from build123d import *

# Parameters (mm, degrees)
ESQUISSE1_R      = 28.5
EXTRUSION1_DEPTH = 5
ESQUISSE2_R      = 7.5
EXTRUSION2_DEPTH = 5
EXTRUSION3_REACH = 43.527
ESQUISSE3_R      = 2.5
ESQUISSE12_W     = 1.25
ESQUISSE12_H     = 28.5


with BuildPart() as part:
    # Esquisse1 → Extrusion1 (new body)
    with BuildSketch(Plane.XY):
        Circle(ESQUISSE1_R)
    extrude(amount=-EXTRUSION1_DEPTH)

    # Esquisse2 → Extrusion2 (add)
    with BuildSketch(Plane.XY):
        Circle(ESQUISSE2_R)
    extrude(amount=EXTRUSION2_DEPTH)

    # Esquisse3 → Extrusion3 (cut, up to next)
    with BuildSketch(Plane.XY.offset(5), mode=Mode.PRIVATE) as extrusion3_sk1:
        Circle(ESQUISSE3_R)
    extrusion3_tool1 = extrude(extrusion3_sk1.sketch, amount=-EXTRUSION3_REACH, mode=Mode.PRIVATE) & part.part
    add(extrusion3_tool1.solids().sort_by_distance((0, 0, 5))[0], mode=Mode.SUBTRACT)

    # Esquisse6 → Enlèvement de matière-Révolution3 (revolve, cut)
    with BuildSketch(Plane(origin=(0, 0, 0), x_dir=(1, 0, 0), z_dir=(0, 1, 0)), mode=Mode.PRIVATE) as enl_vement_de_mati_re_r_volution3_sk:
        with BuildLine():
            Line((-29, 4.5), (-31.449617094, 4.5))
            Line((-31.449617094, 4.5), (-31.449617094, 0.5))
            Line((-31.449617094, 0.5), (-29, 0.5))
            ThreePointArc((-29, 0.5), (-27, 2.5), (-29, 4.5))
        make_face()
    revolve(enl_vement_de_mati_re_r_volution3_sk.sketch.rotate(Axis((0, 0, 5), (0, 0, -1)), 180), axis=Axis((0, 0, 5), (0, 0, -1)), mode=Mode.SUBTRACT)

    # Esquisse12 → Trou taraudé M3x0.55 (revolve, cut)
    with BuildSketch(Plane(origin=(0, 0, 2.5), x_dir=(0, 0, 1), z_dir=(1, 0, 0))):
        with Locations((0.625, 14.25)):
            Rectangle(ESQUISSE12_W, ESQUISSE12_H)
    revolve(axis=Axis((0, 6.35, 2.5), (0, -1, 0)), mode=Mode.SUBTRACT)


solid = part.part
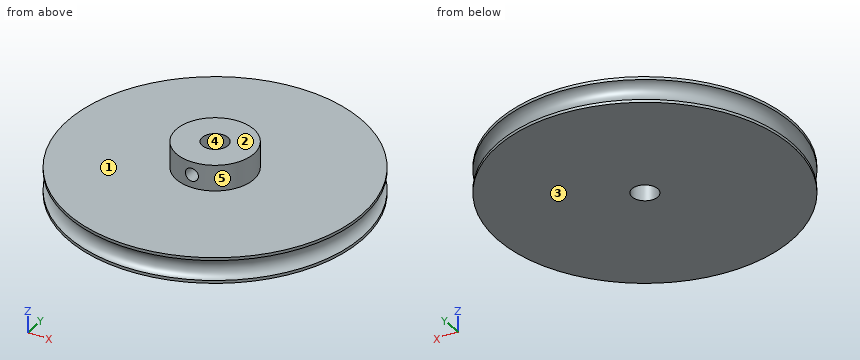
CAD build for the part. Positions are in the model's coordinates, mm. Face numbers are marked on the shaded views. A direction names the side the tool comes from. Round coordinates to 2 decimals unless told otherwise and drop trailing zeros. Loops run counter-clockwise (first coordinate to the right, second up) from the corner with the lowest first, then second, coordinate; pieces in that order, holes last.
(1) Cut at B-B (x = 0). Give the cut face in (y, z).
(2) Drop flat-ended pins along their axis: pin 1 (1.5 mm diameter, centred on x = 16, y = 18.5, fed in from +Z); pin 2 (1.5 mm diameter, centred on x = 0, z = 2.5, fed in from +Y); pin 3 (1.5 mm diameter, centred on y = 8, z = -2, fed in from -X); pin 4 (3 mm diameter, centred on x = 0, y = 0, fed in from -Z). Give the stop position or say it passes through.
(3) Cut at A-A (y = 0). Give the cut face in (x, z).
(4) Which spindle directions (+Z, -Z, +X, -X, +Y, -Y) get a long thin tool onto all of the face, cutting with end or side? Do the marked faces 1 and 2. Say none if no direction does.
(5) Cut at C-C (z = -1.5). Give the cut face in (x, y).
(6) Wall check: line 1 along Z through (x, y) = (0, -5.45); line 2 along Z through (x, y) = (15.5, 21); line 3 along X through (y, z) = (-0.5, -2.25). Give the ranges that are in metal, low to high.
(7) Cut at D-D (z = 2.5). Give the cut face in (x, y), plus the area to 3 significant figures.
(8) Two-plate mould, pull along X, no slides. Class the marked faces 3, 4 and 5: +X half, -X half, draft (parallel to the pull), parting line (faces both ways), or undercut.
Findings below:
1. outline: (-28.5, -5) - (-2.5, -5) - (-2.5, 1.25) - (-7.5, 1.25) - (-7.5, 0) - (-28.5, 0) - (-28.5, -0.56) arc R2 cw to (-28.5, -4.44) - close; (-7.5, 3.75) - (-2.5, 3.75) - (-2.5, 5) - (-7.5, 5) - close; (2.5, -5) - (28.5, -5) - (28.5, -4.44) arc R2 cw to (28.5, -0.56) - (28.5, 0) - (7.5, 0) - (7.5, 5) - (2.5, 5) - close
2. pin 1: stops at z = 0
2. pin 2: stops at y = 7.5
2. pin 3: stops at x = -26.29
2. pin 4: passes through
3. outline: (-28.5, -5) - (-2.5, -5) - (-2.5, 5) - (-7.5, 5) - (-7.5, 0) - (-28.5, 0) - (-28.5, -0.56) arc R2 cw to (-28.5, -4.44) - close; (2.5, -5) - (28.5, -5) - (28.5, -4.44) arc R2 cw to (28.5, -0.56) - (28.5, 0) - (7.5, 0) - (7.5, 5) - (2.5, 5) - close
4. face 1: +Z
4. face 2: +Z, +X, -X, +Y, -Y
5. outline: circle Ø54.54 at (0, 0); hole circle Ø5 at (0, 0)
6. line 1: z = -5 to 1.25, 3.75 to 5
6. line 2: z = -5 to 0
6. line 3: x = -27.01 to -2.45, 2.45 to 27.01
7. outline: (-1.25, -7.4) - (-1.25, -2.17) arc R2.5 cw (long way) to (1.25, -2.17) - (1.25, -7.4) arc R7.5 ccw (long way) to start
7. area: 144 mm2
8. face 3: draft
8. face 4: undercut
8. face 5: parting line
